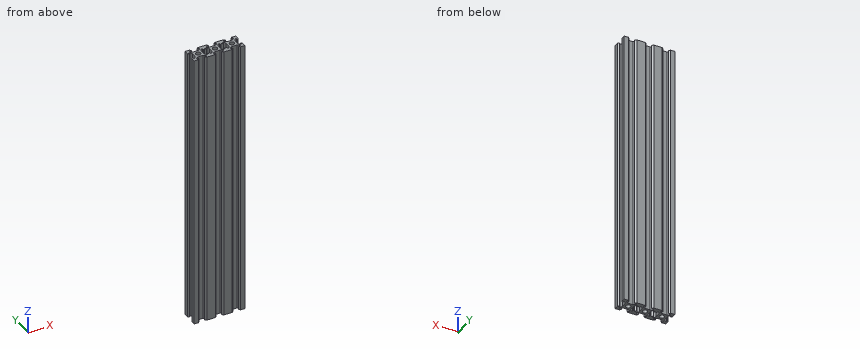
from build123d import *

# Parameters (mm, degrees)
SKETCH1_R           = 4.25
BOSS_EXTRUDE1_DEPTH = 250


with BuildPart() as part:
    # Sketch1 → Boss-Extrude1 (new, symmetric)
    with BuildSketch(Plane.XY):
        Polygon((45, 7.5), (45, 15), (37.5, 15), (35, 12.5), (38.5, 12.5), (38.5, 10), (34.602885683, 7.75), (25.397114317, 7.75), (21.5, 10), (21.5, 12.5), (25, 12.5), (22.5, 15), (7.5, 15), (5, 12.5), (8.5, 12.5), (8.5, 10), (4.602885683, 7.75), (-4.602885683, 7.75), (-8.5, 10), (-8.5, 12.5), (-5, 12.5), (-7.5, 15), (-22.5, 15), (-25, 12.5), (-21.5, 12.5), (-21.5, 10), (-25.397114317, 7.75), (-34.602885683, 7.75), (-38.5, 10), (-38.5, 12.5), (-35, 12.5), (-37.5, 15), (-45, 15), (-45, 7.5), (-42.5, 5), (-42.5, 8.5), (-40, 8.5), (-37.75, 4.602885683), (-37.75, -4.602885683), (-40, -8.5), (-42.5, -8.5), (-42.5, -5), (-45, -7.5), (-45, -15), (-37.5, -15), (-35, -12.5), (-38.5, -12.5), (-38.5, -10), (-34.602885683, -7.75), (-25.397114317, -7.75), (-21.5, -10), (-21.5, -12.5), (-25, -12.5), (-22.5, -15), (-7.5, -15), (-5, -12.5), (-8.5, -12.5), (-8.5, -10), (-4.602885683, -7.75), (4.602885683, -7.75), (8.5, -10), (8.5, -12.5), (5, -12.5), (7.5, -15), (22.5, -15), (25, -12.5), (21.5, -12.5), (21.5, -10), (25.397114317, -7.75), (34.602885683, -7.75), (38.5, -10), (38.5, -12.5), (35, -12.5), (37.5, -15), (45, -15), (45, -7.5), (42.5, -5), (42.5, -8.5), (40, -8.5), (37.75, -4.602885683), (37.75, 4.602885683), (40, 8.5), (42.5, 8.5), (42.5, 5), align=None)
        with Locations((-30, 0)):
            Circle(SKETCH1_R, mode=Mode.SUBTRACT)
        Polygon((-17.5, 8.5), (-17.5, 5), (-15, 7.5), (-12.5, 5), (-12.5, 8.5), (-10, 8.5), (-7.75, 4.602885683), (-7.75, -4.602885683), (-10, -8.5), (-12.5, -8.5), (-12.5, -5), (-15, -7.5), (-17.5, -5), (-17.5, -8.5), (-20, -8.5), (-22.25, -4.602885683), (-22.25, 4.602885683), (-20, 8.5), align=None, mode=Mode.SUBTRACT)
        Circle(SKETCH1_R, mode=Mode.SUBTRACT)
        Polygon((15, 7.5), (17.5, 5), (17.5, 8.5), (20, 8.5), (22.25, 4.602885683), (22.25, -4.602885683), (20, -8.5), (17.5, -8.5), (17.5, -5), (15, -7.5), (12.5, -5), (12.5, -8.5), (10, -8.5), (7.75, -4.602885683), (7.75, 4.602885683), (10, 8.5), (12.5, 8.5), (12.5, 5), align=None, mode=Mode.SUBTRACT)
        with Locations((30, 0)):
            Circle(SKETCH1_R, mode=Mode.SUBTRACT)
    extrude(amount=BOSS_EXTRUDE1_DEPTH, both=True)


solid = part.part
Input: part model. Units: mm. Frame: model coordinates. Coordinates: 2 decimals unless noted, no trailing zeros. Loops run counter-clockwise (first coordinate to the right, second up) from the corner with the lowest first, then second, coordinate; pieces in that order, holes last. Notation, with made-up numbers: (81.5, -7.5) -> (94.5, -7.5) arc R24 cw to (94.5, 15.5) -> close; hole circle Ø1 at (-32, 78). An arc over 180 degrees is marked (long way). Write item = value, one per line. Start each with the question number.
Item 1: Cut plane A-A, the plane y = 0. Return loops of the section in (x, z), plus the area to 3 significant figures.
Item 2: Cut plane B-B, the plane x = 30. Return loops of the section in (y, z), plus the area to 3 significant figures.
Item 3: Material intervals for line 1 (X direction, y = 11, z = 86.5); line 2 (Y direction, x = 0, z = 128); line 3 (Y direction, x = -23, z = 76.5), sorted ascending.
Item 4: Cut plane C-C, the plane z = -12.5. Count the separate pieces of the cut face and the enclosed holes in it, plus the area to 3 significant figures.
Item 5: First-contact query: P1, Ø3, axis at x = -31, z = -6, coming from the +Y side; P2, Ø1.8, axis at x = 6.5, z = -13.5, coming from the +Y side; P3, Ø10, axis at y = -0.5, z = -60, coming from the -X side. Flat tips, straight axial feed; report the tip coordinate or a pass-through.
Ans:
q1.outline = (-37.75, -250) -> (-34.25, -250) -> (-34.25, 250) -> (-37.75, 250) -> close; (-25.75, -250) -> (-22.25, -250) -> (-22.25, 250) -> (-25.75, 250) -> close; (-7.75, -250) -> (-4.25, -250) -> (-4.25, 250) -> (-7.75, 250) -> close; (4.25, -250) -> (7.75, -250) -> (7.75, 250) -> (4.25, 250) -> close; (22.25, -250) -> (25.75, -250) -> (25.75, 250) -> (22.25, 250) -> close; (34.25, -250) -> (37.75, -250) -> (37.75, 250) -> (34.25, 250) -> close
q1.area = 10,500 mm²
q2.outline = (-7.75, -250) -> (-4.25, -250) -> (-4.25, 250) -> (-7.75, 250) -> close; (4.25, -250) -> (7.75, -250) -> (7.75, 250) -> (4.25, 250) -> close
q2.area = 3,500 mm²
q3.line_1 = -45 to -38.5, -21.5 to -8.5, 8.5 to 21.5, 38.5 to 45
q3.line_2 = -7.75 to -4.25, 4.25 to 7.75
q3.line_3 = -14.5 to -12.5, -9.13 to 9.13, 12.5 to 14.5
q4.separate_pieces = 1
q4.enclosed_holes = 5
q4.area = 1,290 mm²
q5.P1 = 7.75
q5.P2 = 14.9
q5.P3 = -43
